Could you check a few things on this drawing? It's one solid part, dimensions in mm from its lowest x, y, z. Give positions to 0.01 mm unless a question says otherwise; leave off trailing zeros. Order: outer loops, then holes, each group sorted by start corner. A loop starts at its lowest first (then second) coordinate and runs counter-clockwise, first axis right, second up. Notation, with made-up numbers: (45.5, 54) -> (65.5, 54) arc R37 ccw to (65.5, 90) -> close; hole circle Ø1 at (71, 41.25). An arc over 180 degrees is marked (long way). Write each question's results on one line, items separated by ' | '.
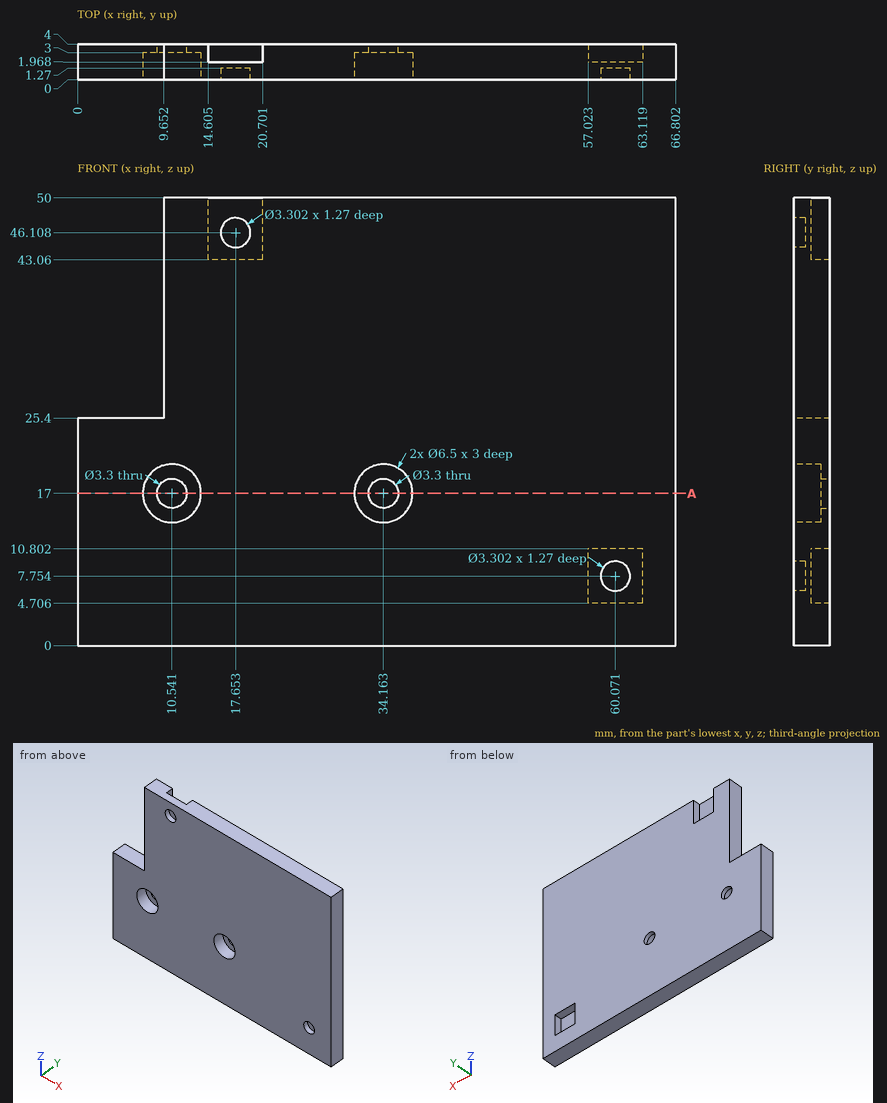
Q1. I need wall thicknesses on line 1 along Z through (x, y) = (60, 1.2) (1 decimal); line 2 along X through (y, z) = (2.45, 7.5); line 3 along Z through (x, y) = (34, 1.55). Which ranges of each line are inside material? Lowest first, please.
Here are the results:
line 1: z = 0 to 6.1, 9.4 to 50 | line 2: x = 0 to 57.02, 63.12 to 66.8 | line 3: z = 0 to 13.75, 20.25 to 50
Q2. I'm going to push flat-ended pins straight in: pin 1 Ø2.5 at (x, z) = (17.5, 46) entering from -Y; pin 2 Ø1 at (x, y) = (18.5, 2.5) entering from +Z; pin 3 Ø1.2 at (x, y) = (6, 2.5) entering from +Z. Where does each tip first touch, or does it pass through?
Here are the results:
pin 1: stops at y = 1.27 | pin 2: stops at z = 43.06 | pin 3: stops at z = 25.4
Q3. Suppose I cut it at A-A on z = 17. Please give me the cut outline in (x, y).
Here are the results:
outline: (0, 0) -> (7.29, 0) -> (7.29, 3) -> (8.89, 3) -> (8.89, 4) -> (0, 4) -> close; (12.19, 3) -> (13.79, 3) -> (13.79, 0) -> (30.91, 0) -> (30.91, 3) -> (32.51, 3) -> (32.51, 4) -> (12.19, 4) -> close; (35.81, 3) -> (37.41, 3) -> (37.41, 0) -> (66.8, 0) -> (66.8, 4) -> (35.81, 4) -> close
